Input: part model. Units: mm. Frame: model coordinates. A direction names the side the tool comes from. Round coordinates to 2 decimals unless told otherwise and drop trailing zeros. Loops run counter-clockwise (first coordinate to the right, second up) from the corner with the lowest first, then second, coordinate; pieces in that order, holes last. Notation, with made-up numbers: (5.5, 40.25) -> (47.5, 40.25) arc R12 cw to (47.5, 44.25) -> close; hole circle Ø11 at (14, 64). An arc over 180 degrees is marked (long way). Answer as a JSON object with one key per item and string values. Group by question number.
Item 1: Set-up query: faces 1 (the flat face through (0, 38.25, 14)), 2 (the flat face through (15.25, 0, 29)). Return all of +Z, -Z, +X, -X, +Y, -Y with unobstructed straight access to the full face (end or side cutting, diameter ignored); none if empty.
Item 2: Section query C-C on y = -6.5. Return loops of the section in (x, z).
Item 3: Draft query along X for faces 3 (the cylindrical face through (9, 34, 10)), 4 (the flat face through (0, 1, 0)), 5 (the cylindrical face through (17.65, -37.68, 14.83)). Return one class per face: released by +X, released by -X, zero draft, split by the parting line, or undercut.
Item 4: Section query B-B on z = 10. Return loops of the section in (x, y) (3 decimals).
Item 5: Pin query (flat end, axial travel): pin 1 (1.8 mm diameter, centred on x = 11.5, y = -31.5, fed in from +Z); pin 2 (2.5 mm diameter, centred on x = -11, y = -31, fed in from +Z). Return the tip coordinate at first contact, or that it passes through.
Item 6: Material intervals for line 1 (Z direction, x = 7.5, y = 34.75); line 2 (X direction, y = 36.25, z = 10); line 3 (X direction, y = 7, z = 27.5), sorted ascending. Write a range as [from, to].
Item 7: Section query D-D on x = -7.5. Return loops of the section in (y, z).
Item 8: Section query A-A on z = 15. Return loops of the section in (x, y) (3 decimals).
from build123d import *

# Parameters (mm, degrees)
BASE_SKETCH_W           = 36.5
BASE_SKETCH_H           = 76.5
BASE_SKETCH_W_2         = 30.5
BASE_SKETCH_H_2         = 70.5
BASE_SKETCH_R           = 1.475
BOSS_EXTRUDE1_DEPTH     = 3
BOSS_EXTRUDE2_START     = 3
BASE_SKETCH_8_W         = 36.5
BASE_SKETCH_8_H         = 76.5
BASE_SKETCH_8_W_2       = 30.5
BASE_SKETCH_8_H_2       = 70.5
BASE_SKETCH_8_R         = 1.475
BOSS_EXTRUDE2_DEPTH     = 24
BOSS_EXTRUDE3_START     = 27
BASE_SKETCH_9_W         = 36.5
BASE_SKETCH_9_H         = 76.5
BASE_SKETCH_9_W_2       = 30.5
BASE_SKETCH_9_H_2       = 70.5
BOSS_EXTRUDE3_DEPTH     = 3.25
FILLET1_R               = 2
FILLET2_R               = 1
CHAMFER1_SIZE           = 1
CUT_EXTRUDE1_REACH      = 86.264
CUT_EXTRUDE1_END_RADIUS = 14
SKETCH1_R               = 1.5


with BuildPart() as part:
    # Base_Sketch → Boss-Extrude1 (new body)
    # profile 1 of 7: a face of its own
    with BuildSketch(Plane.XY):
        Rectangle(BASE_SKETCH_W, BASE_SKETCH_H)
        Rectangle(BASE_SKETCH_W_2, BASE_SKETCH_H_2, mode=Mode.SUBTRACT)
    # profile 2 of 7: a face of its own
    with BuildSketch(Plane.XY):
        Rectangle(BASE_SKETCH_W_2, BASE_SKETCH_H_2)
        with Locations((-11.5, -31.5)):
            Circle(BASE_SKETCH_R, mode=Mode.SUBTRACT)
        with Locations((11.5, -31.5)):
            Circle(BASE_SKETCH_R, mode=Mode.SUBTRACT)
        with Locations((11.5, 31.5)):
            Circle(BASE_SKETCH_R, mode=Mode.SUBTRACT)
        with Locations((-11.5, 31.5)):
            Circle(BASE_SKETCH_R, mode=Mode.SUBTRACT)
        with BuildLine():
            ThreePointArc((-14, -19), (0, -33), (14, -19))
            Line((14, -19), (14, 19))
            ThreePointArc((14, 19), (0, 33), (-14, 19))
            Line((-14, 19), (-14, -19))
        make_face(mode=Mode.SUBTRACT)
    # profile 3 of 7: a face of its own
    with BuildSketch(Plane.XY):
        with Locations((-11.5, -31.5)):
            Circle(BASE_SKETCH_R)
    # profile 4 of 7: a face of its own
    with BuildSketch(Plane.XY):
        with Locations((11.5, -31.5)):
            Circle(BASE_SKETCH_R)
    # profile 5 of 7: a face of its own
    with BuildSketch(Plane.XY):
        with Locations((11.5, 31.5)):
            Circle(BASE_SKETCH_R)
    # profile 6 of 7: a face of its own
    with BuildSketch(Plane.XY):
        with Locations((-11.5, 31.5)):
            Circle(BASE_SKETCH_R)
    # profile 7 of 7: a face of its own
    with BuildSketch(Plane.XY):
        with BuildLine():
            Line((-14, 19), (-14, -19))
            ThreePointArc((-14, -19), (0, -33), (14, -19))
            Line((14, -19), (14, 19))
            ThreePointArc((14, 19), (0, 33), (-14, 19))
        make_face()
    extrude(amount=BOSS_EXTRUDE1_DEPTH)

    # Base_Sketch<8> → Boss-Extrude2 (add)
    # profile 1 of 2: a face of its own
    with BuildSketch(Plane.XY.offset(BOSS_EXTRUDE2_START)):
        Rectangle(BASE_SKETCH_8_W, BASE_SKETCH_8_H)
        Rectangle(BASE_SKETCH_8_W_2, BASE_SKETCH_8_H_2, mode=Mode.SUBTRACT)
    # profile 2 of 2: a face of its own
    with BuildSketch(Plane.XY.offset(BOSS_EXTRUDE2_START)):
        Rectangle(BASE_SKETCH_8_W_2, BASE_SKETCH_8_H_2)
        with Locations((-11.5, -31.5)):
            Circle(BASE_SKETCH_8_R, mode=Mode.SUBTRACT)
        with Locations((11.5, -31.5)):
            Circle(BASE_SKETCH_8_R, mode=Mode.SUBTRACT)
        with Locations((11.5, 31.5)):
            Circle(BASE_SKETCH_8_R, mode=Mode.SUBTRACT)
        with Locations((-11.5, 31.5)):
            Circle(BASE_SKETCH_8_R, mode=Mode.SUBTRACT)
        with BuildLine():
            ThreePointArc((-14, -19), (0, -33), (14, -19))
            Line((14, -19), (14, 19))
            ThreePointArc((14, 19), (0, 33), (-14, 19))
            Line((-14, 19), (-14, -19))
        make_face(mode=Mode.SUBTRACT)
    extrude(amount=BOSS_EXTRUDE2_DEPTH)

    # Base_Sketch<9> → Boss-Extrude3 (add)
    with BuildSketch(Plane.XY.offset(BOSS_EXTRUDE3_START)):
        Rectangle(BASE_SKETCH_9_W, BASE_SKETCH_9_H)
        Rectangle(BASE_SKETCH_9_W_2, BASE_SKETCH_9_H_2, mode=Mode.SUBTRACT)
    extrude(amount=BOSS_EXTRUDE3_DEPTH)

    # Fillet1
    fillet1_edges = [part.edges().sort_by_distance(p)[0] for p in [
        (-18.25, 38.25, 15.125),
        (18.25, 38.25, 15.125),
        (18.25, -38.25, 15.125),
        (-18.25, -38.25, 15.125),
    ]]
    fillet(fillet1_edges, radius=FILLET1_R)

    # Fillet2
    fillet2_edges = [part.edges().sort_by_distance(p)[0] for p in [
        (-15.25, 35.25, 28.625),
        (-15.25, -35.25, 28.625),
        (15.25, -35.25, 28.625),
        (15.25, 35.25, 28.625),
    ]]
    fillet(fillet2_edges, radius=FILLET2_R)

    # Chamfer1
    chamfer1_edges = [part.edges().sort_by_distance(p)[0] for p in [
        (0, -38.25, 30.25),
        (-18.25, 0, 30.25),
        (18.25, 0, 30.25),
        (0, 38.25, 30.25),
        (17.664213562, -37.664213562, 30.25),
        (17.664213562, 37.664213562, 30.25),
        (-17.664213562, 37.664213562, 30.25),
        (-17.664213562, -37.664213562, 30.25),
    ]]
    chamfer(chamfer1_edges, length=CHAMFER1_SIZE)

    # Cut-Extrude1: up to this cylinder (the profile starts outside it)
    cut_extrude1_end = Plane(origin=(0, 19, 10), z_dir=(0, 0, -1)) * Cylinder(CUT_EXTRUDE1_END_RADIUS, 201.528, mode=Mode.PRIVATE)
    # Sketch1 → Cut-Extrude1 (cut, up to the surface)
    with BuildSketch(Plane(origin=(0, 38.25, 0), x_dir=(1, 0, 0), z_dir=(0, 1, 0)), mode=Mode.PRIVATE) as cut_extrude1_sk1:
        with Locations(Location((-7.5, -10, 0), (0, 0, 270))):
            Circle(SKETCH1_R)
    cut_extrude1_tool1 = extrude(cut_extrude1_sk1.sketch, amount=-CUT_EXTRUDE1_REACH, mode=Mode.PRIVATE) - cut_extrude1_end
    add(cut_extrude1_tool1.solids().sort_by_distance((-7.5, 38.25, 10))[0], mode=Mode.SUBTRACT)
    # Sketch1 → Cut-Extrude1 (cut, up to the surface)
    with BuildSketch(Plane(origin=(0, 38.25, 0), x_dir=(1, 0, 0), z_dir=(0, 1, 0)), mode=Mode.PRIVATE) as cut_extrude1_sk2:
        with Locations(Location((7.5, -10, 0), (0, 0, 270))):
            Circle(SKETCH1_R)
    cut_extrude1_tool2 = extrude(cut_extrude1_sk2.sketch, amount=-CUT_EXTRUDE1_REACH, mode=Mode.PRIVATE) - cut_extrude1_end
    add(cut_extrude1_tool2.solids().sort_by_distance((7.5, 38.25, 10))[0], mode=Mode.SUBTRACT)


solid = part.part
Solved:
{
 "1": {"face 1": "+Z, -Z, +X, -X, +Y", "face 2": "+Z"},
 "2": {"outline": "(-18.25, 0) -> (18.25, 0) -> (18.25, 29.25) -> (17.25, 30.25) -> (15.25, 30.25) -> (15.25, 27) -> (14, 27) -> (14, 3) -> (-14, 3) -> (-14, 27) -> (-15.25, 27) -> (-15.25, 30.25) -> (-17.25, 30.25) -> (-18.25, 29.25) -> close"},
 "3": {"face 3": "undercut", "face 4": "zero draft", "face 5": "released by +X"},
 "4": {"outline": "(-18.25, -36.25) arc R2 ccw to (-16.25, -38.25) -> (16.25, -38.25) arc R2 ccw to (18.25, -36.25) -> (18.25, 36.25) arc R2 ccw to (16.25, 38.25) -> (9, 38.25) -> (9, 29.724) arc R14 cw to (14, 19) -> (14, -19) arc R14 cw to (-14, -19) -> (-14, 19) arc R14 cw to (-9, 29.724) -> (-9, 38.25) -> (-16.25, 38.25) arc R2 ccw to (-18.25, 36.25) -> close; (-6, 31.649) arc R14 cw to (6, 31.649) -> (6, 38.25) -> (-6, 38.25) -> close; hole circle Ø2.95 at (-11.5, -31.5); hole circle Ø2.95 at (-11.5, 31.5); hole circle Ø2.95 at (11.5, -31.5); hole circle Ø2.95 at (11.5, 31.5)"},
 "5": {"pin 1": "z = 3", "pin 2": "z = 27"},
 "6": {"line 1": "[0, 8.5], [11.5, 27]", "line 2": "[-18.25, -9], [-6, 6], [9, 18.25]", "line 3": "[-18.25, -15.25], [15.25, 18.25]"},
 "7": {"outline": "(-38.25, 0) -> (38.25, 0) -> (38.25, 8.5) -> (30.82, 8.5) -> (30.82, 3) -> (-30.82, 3) -> (-30.82, 27) -> (-35.25, 27) -> (-35.25, 30.25) -> (-37.25, 30.25) -> (-38.25, 29.25) -> close; (30.82, 11.5) -> (38.25, 11.5) -> (38.25, 29.25) -> (37.25, 30.25) -> (35.25, 30.25) -> (35.25, 27) -> (30.82, 27) -> close"},
 "8": {"outline": "(-18.25, -36.25) arc R2 ccw to (-16.25, -38.25) -> (16.25, -38.25) arc R2 ccw to (18.25, -36.25) -> (18.25, 36.25) arc R2 ccw to (16.25, 38.25) -> (-16.25, 38.25) arc R2 ccw to (-18.25, 36.25) -> close; hole (-14, -19) arc R14 ccw to (14, -19) -> (14, 19) arc R14 ccw to (-14, 19) -> close; hole circle Ø2.95 at (-11.5, -31.5); hole circle Ø2.95 at (-11.5, 31.5); hole circle Ø2.95 at (11.5, -31.5); hole circle Ø2.95 at (11.5, 31.5)"}
}
